```python
from build123d import *

# Parameters (mm, degrees)
F0_R      = 40
F1_DEPTH  = 13
F1_TAPER  = 65
F2_DEPTH  = 2
F2_FACE_R = 12.1214100334
F3_DEPTH  = 13
F3_TAPER  = -65
F4_R      = 11
F5_DEPTH  = 5
F6_R      = 3
F7_DEPTH  = 50
F6_R_2    = 1.25
F8_DEPTH  = 20
F9_R      = 13.260393294
F9_R_2    = 3
F10_DEPTH = 5


with BuildPart() as f1:
    # F0 (on Top) → F1 (new body)
    with BuildSketch(Plane.XY):
        with Locations((-0.3933568078, 0)):
            Circle(F0_R)
    extrude(amount=F1_DEPTH, taper=F1_TAPER)

    # F2 (add): a face of the model
    f2_faces = [f1.faces().sort_by_distance(p)[0] for p in [
        (-0.3933568078, 0, 13),
    ]]
    extrude(f2_faces, amount=F2_DEPTH)

    # F2_face (on face) → F3 (join)
    with BuildSketch(Plane(origin=(-0.3933568078, 0, 15), x_dir=(1, 0, 0), z_dir=(0, 0, 1))):
        Circle(F2_FACE_R)
    extrude(amount=F3_DEPTH, taper=F3_TAPER)

    # F4 (on face) → F5 (cut)
    with BuildSketch(Plane.XY.offset(28)):
        Circle(F4_R)
    extrude(amount=-F5_DEPTH, mode=Mode.SUBTRACT)

    # F6 (on face) → F7 (cut)
    with BuildSketch(Plane.XY.offset(23)):
        Circle(F6_R)
    extrude(amount=-F7_DEPTH, mode=Mode.SUBTRACT)

    # F6 (on face) → F8 (cut)
    with BuildSketch(Plane.XY.offset(23)):
        with Locations((0, 7.25)):
            Circle(F6_R_2)
        with Locations((7.25, 0)):
            Circle(F6_R_2)
        with Locations((0, -7.25)):
            Circle(F6_R_2)
        with Locations((-7.25, 0)):
            Circle(F6_R_2)
    extrude(amount=-F8_DEPTH, mode=Mode.SUBTRACT)

    # F9 (on face) → F10 (cut)
    with BuildSketch(Plane(origin=(0, 0, 0), x_dir=(1, 0, 0), z_dir=(0, 0, -1))):
        Circle(F9_R)
        Circle(F9_R_2, mode=Mode.SUBTRACT)
    extrude(amount=-F10_DEPTH, mode=Mode.SUBTRACT)


solid = f1.part
```
The listing builds one solid part. Answer for the finished solid, in the listing's coordinates (mm). A direction names the side the tool comes from. Round coordinates to 2 decimals unless told otherwise and drop trailing zeros. Loops run counter-clockwise (first coordinate to the right, second up) from the corner with the lowest first, then second, coordinate; pieces in that order, holes last. Notation, with made-up numbers: (54, -3.5) - (90, -3.5) arc R18 cw to (90, 22.5) - close; hole circle Ø9 at (43.5, 17). An arc over 180 degrees is marked (long way). Return JSON: item names as keys, results as strings. Group by question number.
1. The mould has two halves that part along X. Classify faces 4 (the cylindrical face through (-9.33, -8.19, 13.99)), 5 (the flat face through (8, -8, 28)), 6 (the flat face through (3, 3, 5)), 7 (the cylindrical face through (-10.5, 8.1, 2.5)): pulls with the +X half, pulls with the -X half, needs draft (parallel to the pull), parting line crosses it, or undercut.
2. The part is cut by section B-B on z = 21.5. Determine the outline of the cut face in (x, y).
3. The part is cut by section A-A on y = 0. State how many separate pieces and enclosed holes the cut face has, then the cut area to 3 significant figures.
4. The part is cut by section C-C on z = 2. Determine the outline of the cut face in (x, y), then the cut area to 3 significant figures.
5. The part is cut by section D-D on z = 11.75. Determine the outline of the cut face in (x, y).
6. Consider probe 1 along Y at (x, z) = (0, 10.75); probe 2 along Z at (x, y) = (-10, -2.5); probe 3 along Z at (x, y) = (-13.5, -1.5). Determine where each line is inside the solid, lowest interval first.
7. Each of these flat-tipped pins is pushed along its axis until it touches: P1, Ø3, axis at x = -7.25, y = 0, coming from the +Z side; P2, Ø1.5, axis at x = -5.5, z = 19.5, coming from the +Y side; P3, Ø10, axis at y = 17, z = 6.5, coming from the -X side. Where does it stop, or does it pass through?
8. Which of the six approach directions +Z, -Z, +X, -X, +Y, -Y give full straight-line access (tool end or side, diameter ignored) to faces 1 (the flat face through (2.3, -2.3, 23)), 2 (the conical face through (5.82, -11.95, 12.37)), 3 (the cylindrical face through (-3, 0, 14))?
Resolved:
{
 "1": {"face 4": "parting line crosses it", "face 5": "needs draft", "face 6": "undercut", "face 7": "undercut"},
 "2": {"outline": "circle Ø52.12 at (-0.39, 0); hole circle Ø2.5 at (-7.25, 0); hole circle Ø6 at (0, 0); hole circle Ø2.5 at (0, -7.25); hole circle Ø2.5 at (0, 7.25); hole circle Ø2.5 at (7.25, 0)"},
 "3": {"separate pieces": "4", "enclosed holes": "0", "area": "963 mm²"},
 "4": {"outline": "circle Ø71.42 at (-0.39, 0); hole circle Ø26.52 at (0, 0)", "area": "3,450 mm²"},
 "5": {"outline": "circle Ø29.6 at (-0.39, 0); hole circle Ø2.5 at (-7.25, 0); hole circle Ø6 at (0, 0); hole circle Ø2.5 at (0, -7.25); hole circle Ø2.5 at (0, 7.25); hole circle Ø2.5 at (7.25, 0)"},
 "6": {"probe 1": "y = -16.94 to -8.5, -6 to -3, 3 to 6, 8.5 to 16.94", "probe 2": "z = 5 to 23", "probe 3": "z = 0 to 12.5, 15.5 to 28"},
 "7": {"P1": "stops at z = 23", "P2": "stops at y = 22.82", "P3": "stops at x = -33.27"},
 "8": {"face 1": "+Z", "face 2": "none", "face 3": "+Z, -Z"}
}
